Build history of the part. All positions in model axes, mm. A direction names the side the tool comes from. Give positions to 0.01 mm unless a question says otherwise; leave off trailing zeros. Order: outer loops, then holes, each group sorted by start corner. A loop starts at its lowest first (then second) coordinate and runs counter-clockwise, first axis right, second up. Notation, with made-up numbers: (-16.5, 83) - (-0.5, 83) arc R31 cw to (-0.5, 107) - close; hole circle Ø11 at (38.25, 75.5). An arc over 180 degrees is marked (long way). Use a Markdown table: item, result.
from build123d import *

# Parameters (mm, degrees)
SKETCH_1_W           = 90
SKETCH_1_H           = 50
EXTRUDE_1_DEPTH      = 10
CUT_EXTRUDE_2_DEPTH  = 5
SKETCH_7_R           = 1.6
CUT_EXTRUDE_3_DEPTH  = 10
MIRROR_3_DEPTH       = 10
MIRROR_START         = 5
MIRROR_3_2_OUTLINE_R = 1.6
MIRROR_3_2_DEPTH     = 5
SKETCH_8_R           = 5
EXTRUDE_2_DEPTH      = 30
SKETCH_10_W          = 35
SKETCH_10_H          = 20.2
EXTRUDE_6_DEPTH      = 5
SKETCH_11_W          = 102.2
SKETCH_11_H          = 51.5
CUT_EXTRUDE_4_DEPTH  = 6
SKETCH_12_W          = 7.5
SKETCH_12_H          = 13.7
CUT_EXTRUDE_5_DEPTH  = 50
FILLET_2_R           = 5
CUT_EXTRUDE_6_DEPTH  = 15
CUT_EXTRUDE_7_DEPTH  = 10
SKETCH_15_R          = 5
EXTRUDE_7_DEPTH      = 10
SKETCH_16_R          = 2
CUT_EXTRUDE_8_DEPTH  = 10
SKETCH_17_R          = 1.6
CUT_EXTRUDE_9_DEPTH  = 10


# Read off the part's stored shape, not the designer's step: Зеркальное отражение3
with BuildPart() as part:
    # Эскиз1 → Бобышка-Вытянуть1 (new body)
    with BuildSketch(Plane(origin=(0, 0, 0), x_dir=(1, 0, 0), z_dir=(0, 1, 0))):
        with Locations((4.158751696, -0.305291723)):
            Rectangle(SKETCH_1_W, SKETCH_1_H)
    extrude(amount=EXTRUDE_1_DEPTH)

    # Эскиз2 → Вырез-Вытянуть2 (cut)
    with BuildSketch(Plane.XZ):
        Polygon((-40.841248304, 14.557268649), (-23.163578774, -3.12040088), (-12.4155557, 7.627622194), (-30.09322523, 25.305291723), (-40.841248304, 25.305291723), align=None)
    extrude(amount=-CUT_EXTRUDE_2_DEPTH, mode=Mode.SUBTRACT)

    # Эскиз7 → Вырез-Вытянуть3 (cut)
    with BuildSketch(Plane.XZ.offset(-5)):
        with Locations(Location((-31.931702861, 16.39574628, 0), (0, 0, 270))):
            Circle(SKETCH_7_R)
        with Locations(Location((-23.446421487, 7.910464906, 0), (0, 0, 270))):
            Circle(SKETCH_7_R)
    extrude(amount=-CUT_EXTRUDE_3_DEPTH, mode=Mode.SUBTRACT)

    # Зеркальное отражение3 outline → Зеркальное отражение3 (add)
    with BuildSketch(Plane(origin=(0, 0, 0), x_dir=(1, 0, 0), z_dir=(0, 1, 0))):
        Polygon((-40.841248304, 63.946685203), (-40.841248304, 24.694708277), (49.158751696, 24.694708277), (49.158751696, -25.305291723), (128.410728622, -25.305291723), (110.733059092, -7.627622194), (121.481082166, 3.12040088), (139.158751696, -14.557268649), (139.158751696, 63.946685203), (121.481082166, 46.269015673), (110.733059092, 57.017038747), (128.410728622, 74.694708277), (-30.09322523, 74.694708277), (-12.4155557, 57.017038747), (-23.163578774, 46.269015673), align=None)
    extrude(amount=MIRROR_3_DEPTH)

    # Mirror 3 2 outline → Mirror 3 2 (add)
    # profile 1 of 3: a face of its own
    with BuildSketch(Plane(origin=(0, 0, 0), x_dir=(1, 0, 0), z_dir=(0, 1, 0)).offset(MIRROR_START)):
        Polygon((-40.841248304, 74.694708277), (-40.841248304, 63.946685203), (-23.163578774, 46.269015673), (-12.4155557, 57.017038747), (-30.09322523, 74.694708277), align=None)
        with Locations((-23.446421487, 57.29988146)):
            Circle(MIRROR_3_2_OUTLINE_R, mode=Mode.SUBTRACT)
        with Locations((-31.931702861, 65.785162834)):
            Circle(MIRROR_3_2_OUTLINE_R, mode=Mode.SUBTRACT)
    # profile 2 of 3: a face of its own
    with BuildSketch(Plane(origin=(0, 0, 0), x_dir=(1, 0, 0), z_dir=(0, 1, 0)).offset(MIRROR_START)):
        Polygon((110.733059092, -7.627622194), (128.410728622, -25.305291723), (139.158751696, -25.305291723), (139.158751696, -14.557268649), (121.481082166, 3.12040088), align=None)
        with Locations((130.249206253, -16.39574628)):
            Circle(MIRROR_3_2_OUTLINE_R, mode=Mode.SUBTRACT)
        with Locations((121.763924879, -7.910464906)):
            Circle(MIRROR_3_2_OUTLINE_R, mode=Mode.SUBTRACT)
    # profile 3 of 3: a face of its own
    with BuildSketch(Plane(origin=(0, 0, 0), x_dir=(1, 0, 0), z_dir=(0, 1, 0)).offset(MIRROR_START)):
        Polygon((139.158751696, 74.694708277), (128.410728622, 74.694708277), (110.733059092, 57.017038747), (121.481082166, 46.269015673), (139.158751696, 63.946685203), align=None)
        with Locations((121.763924879, 57.29988146)):
            Circle(MIRROR_3_2_OUTLINE_R, mode=Mode.SUBTRACT)
        with Locations((130.249206253, 65.785162834)):
            Circle(MIRROR_3_2_OUTLINE_R, mode=Mode.SUBTRACT)
    extrude(amount=MIRROR_3_2_DEPTH)

    # Эскиз8 → Бобышка-Вытянуть2 (add)
    with BuildSketch(Plane(origin=(0, 10, 0), x_dir=(1, 0, 0), z_dir=(0, 1, 0))):
        with Locations(Location((49.158751696, 46.794708277, 0), (0, 0, 90))):
            Circle(SKETCH_8_R)
        with Locations(Location((94.158751696, 46.794708277, 0), (0, 0, 90))):
            Circle(SKETCH_8_R)
        with Locations(Location((94.158751696, 2.594708277, 0), (0, 0, 90))):
            Circle(SKETCH_8_R)
        with Locations(Location((4.158751696, 2.594708277, 0), (0, 0, 90))):
            Circle(SKETCH_8_R)
        with Locations(Location((49.158751696, 2.594708277, 0), (0, 0, 90))):
            Circle(SKETCH_8_R)
        with Locations(Location((4.158751696, 46.794708277, 0), (0, 0, 90))):
            Circle(SKETCH_8_R)
    extrude(amount=EXTRUDE_2_DEPTH)

    # Эскиз10 → Бобышка-Вытянуть6 (add)
    with BuildSketch(Plane(origin=(0, 40, 0), x_dir=(1, 0, 0), z_dir=(0, 1, 0))):
        Polygon((9.158751696, 51.794708277), (9.158751696, 39.794708277), (44.158751696, 39.794708277), (44.158751696, 51.794708277), (54.158751696, 51.794708277), (54.158751696, 39.794708277), (89.158751696, 39.794708277), (89.158751696, 51.794708277), (99.158751696, 51.794708277), (99.158751696, -2.405291723), (89.158751696, -2.405291723), (89.158751696, 9.594708277), (54.158751696, 9.594708277), (54.158751696, -2.405291723), (44.158751696, -2.405291723), (44.158751696, 9.594708277), (9.158751696, 9.594708277), (9.158751696, -2.405291723), (-0.841248304, -2.405291723), (-0.841248304, 51.794708277), align=None)
        with Locations((26.658751696, 24.694708277)):
            Rectangle(SKETCH_10_W, SKETCH_10_H, mode=Mode.SUBTRACT)
        with Locations((71.658751696, 24.694708277)):
            Rectangle(SKETCH_10_W, SKETCH_10_H, mode=Mode.SUBTRACT)
    extrude(amount=EXTRUDE_6_DEPTH)

    # Эскиз11 → Вырез-Вытянуть4 (cut)
    with BuildSketch(Plane(origin=(0, 0, 0), x_dir=(-1, 0, 0), z_dir=(0, -1, 0))):
        with Locations((-47.698520167, 25.294708277)):
            Rectangle(SKETCH_11_W, SKETCH_11_H)
    extrude(amount=-CUT_EXTRUDE_4_DEPTH, mode=Mode.SUBTRACT)

    # Эскиз12 → Вырез-Вытянуть5 (cut)
    with BuildSketch(Plane(origin=(0, 10, 0), x_dir=(1, 0, 0), z_dir=(0, 1, 0))):
        with Locations((108.408751696, 24.844708277)):
            Rectangle(SKETCH_12_W, SKETCH_12_H)
    extrude(amount=-CUT_EXTRUDE_5_DEPTH, mode=Mode.SUBTRACT)

    # Скругление2
    fillet_2_edges = [part.edges().sort_by_distance(p)[0] for p in [
        (54.158751696, 42.5, -9.594708277),
        (9.158751696, 42.5, -9.594708277),
        (-0.841248304, 42.5, 2.405291723),
        (9.158751696, 42.5, 2.405291723),
        (44.158751696, 42.5, -9.594708277),
        (54.158751696, 42.5, 2.405291723),
        (44.158751696, 42.5, 2.405291723),
        (89.158751696, 42.5, -9.594708277),
        (89.158751696, 42.5, 2.405291723),
        (99.158751696, 42.5, 2.405291723),
        (54.158751696, 42.5, -39.794708277),
        (9.158751696, 42.5, -39.794708277),
        (44.158751696, 42.5, -39.794708277),
        (99.158751696, 42.5, -51.794708277),
        (89.158751696, 42.5, -39.794708277),
        (89.158751696, 42.5, -51.794708277),
        (54.158751696, 42.5, -51.794708277),
        (44.158751696, 42.5, -51.794708277),
        (9.158751696, 42.5, -51.794708277),
        (-0.841248304, 42.5, -51.794708277),
    ]]
    fillet(fillet_2_edges, radius=FILLET_2_R - 0.0001)  # a hair under: the kernel refuses the full size

    # Эскиз13 → Вырез-Вытянуть6 (cut)
    with BuildSketch(Plane.XZ):
        Polygon((-15.09322523, 25.305291723), (2.5844443, 7.627622194), (95.733059092, 7.627622194), (113.410728622, 25.305291723), align=None)
        Polygon((-40.841248304, -0.442731351), (-23.163578774, -18.12040088), (-23.163578774, -31.269015673), (-40.841248304, -48.946685203), align=None)
        Polygon((-15.09322523, -74.694708277), (2.5844443, -57.017038747), (95.733059092, -57.017038747), (113.410728622, -74.694708277), align=None)
        Polygon((139.158751696, -0.442731351), (121.481082166, -18.12040088), (121.481082166, -31.269015673), (139.158751696, -48.946685203), align=None)
    extrude(amount=-CUT_EXTRUDE_6_DEPTH, mode=Mode.SUBTRACT)

    # Эскиз14 → Вырез-Вытянуть7 (cut)
    with BuildSketch(Plane.XZ.offset(-6)):
        Polygon((4.598520167, -9.023164144), (4.598520167, -40.56625241), (41.357986916, -24.794708277), align=None)
        Polygon((13.833681258, -7.544708277), (47.698520167, -22.074320609), (81.563359076, -7.544708277), align=None)
        Polygon((13.833681258, -42.044708277), (47.698520167, -27.515095944), (81.563359076, -42.044708277), align=None)
        Polygon((54.039053419, -24.794708277), (90.798520167, -40.56625241), (90.798520167, -9.023164144), align=None)
    extrude(amount=-CUT_EXTRUDE_7_DEPTH, mode=Mode.SUBTRACT)

    # Эскиз15 → Бобышка-Вытянуть7 (add)
    with BuildSketch(Plane.XZ):
        with Locations((49.158751696, 7.627622194)):
            Circle(SKETCH_15_R)
        with Locations((-23.163578774, -24.694708277)):
            Circle(SKETCH_15_R)
        with Locations((121.481082166, -24.694708277)):
            Circle(SKETCH_15_R)
        with Locations((49.158751696, -57.017038747)):
            Circle(SKETCH_15_R)
    extrude(amount=-EXTRUDE_7_DEPTH)

    # Эскиз16 → Вырез-Вытянуть8 (cut)
    with BuildSketch(Plane.XZ):
        with Locations(Location((49.158751696, 7.627622194, 0), (0, 0, 270))):
            Circle(SKETCH_16_R)
        with Locations(Location((-23.163578774, -24.694708277, 0), (0, 0, 270))):
            Circle(SKETCH_16_R)
        with Locations(Location((121.481082166, -24.694708277, 0), (0, 0, 270))):
            Circle(SKETCH_16_R)
        with Locations(Location((49.158751696, -57.017038747, 0), (0, 0, 270))):
            Circle(SKETCH_16_R)
    extrude(amount=-CUT_EXTRUDE_8_DEPTH, mode=Mode.SUBTRACT)

    # Эскиз17 → Вырез-Вытянуть9 (cut)
    with BuildSketch(Plane(origin=(0, 45, 0), x_dir=(1, 0, 0), z_dir=(0, 1, 0))):
        with Locations(Location((4.158751696, 34.74175422, 0), (0, 0, 270))):
            Circle(SKETCH_17_R)
        with Locations(Location((94.158751696, 34.794708277, 0), (0, 0, 270))):
            Circle(SKETCH_17_R)
        with Locations(Location((94.158751696, 14.594708277, 0), (0, 0, 270))):
            Circle(SKETCH_17_R)
        with Locations(Location((4.158751696, 14.594708277, 0), (0, 0, 270))):
            Circle(SKETCH_17_R)
    extrude(amount=-CUT_EXTRUDE_9_DEPTH, mode=Mode.SUBTRACT)


solid = part.part
1) Two-plate mould, pull along Y, no slides. Class faces 5 (the flat face through (-31.879, 2.465, -54.984)), 6 (the flat face through (-27, 5, 11)), 7 (the flat face through (50, 40, -25)): +Y half, -Y half, draft (parallel to the pull), parting line (faces both ways), or undercut.
Computed:
| item | result |
|---|---|
| face 5 | draft |
| face 6 | -Y half |
| face 7 | undercut |
2) Slice it at A-A (x = 56.5). Write the cut outline in (y, z), and give its area (3 significant figures).
Computed:
| item | result |
|---|---|
| outline | (0, -57.02) - (10, -57.02) - (10, -42.04) - (6, -42.04) - (6, -51.04) - (0, -51.04) - close; (0, 0.46) - (6, 0.46) - (6, -7.54) - (10, -7.54) - (10, 7.63) - (0, 7.63) - close; (6, -31.29) - (10, -31.29) - (10, -25.85) - (6, -25.85) - close; (6, -23.74) - (10, -23.74) - (10, -18.3) - (6, -18.3) - close; (40, -40.56) - (45, -40.56) - (45, -34.79) - (40, -34.79) - close; (40, -14.59) - (45, -14.59) - (45, -8.83) - (40, -8.83) - close |
| area | 301 mm² |
3) Wall check: line 1 (Z direction, x = 71, y = 9); line 2 (X direction, y = 12, z = -3); line 3 (Z direction, x = -26.5, y = 7). Give the ranges that are in metal, low to high. Write a range as from..to.
Computed:
| item | result |
|---|---|
| line 1 | z = -57.02..-42.04, -37.51..-32.07, -17.52..-12.08, -7.54..7.63 |
| line 2 | x = -0.82..9.14, 44.18..54.14, 89.18..99.14 |
| line 3 | z = -74.69..-34.61, -28.42..-20.97, -14.78..25.31 |
4) Slice it at B-B (y = 27). Write the cut outline in (x, z).
Computed:
| item | result |
|---|---|
| outline | circle Ø10 at (4.16, -46.79); circle Ø10 at (4.16, -2.59); circle Ø10 at (49.16, -46.79); circle Ø10 at (49.16, -2.59); circle Ø10 at (94.16, -46.79); circle Ø10 at (94.16, -2.59) |
5) Pin check, flat tips, straight feed: P1, Ø8, axis at y = 2.5, z = -27.5, coming from the -X side; P2, Ø6.5, axis at x = 58, y = 3.5, coming from the +Z side; P3, Ø1.5, axis at x = 96, z = -1.5, coming from the -Y side. Stop position of each tip, or through.
Computed:
| item | result |
|---|---|
| P1 | stops at x = -28.16 |
| P2 | stops at z = 7.63 |
| P3 | stops at y = 6 |
6) Tool access for faces 1 (the flat face through (-17.71, 2.46, -51.72)), 2 (the cylindrical face through (42.655, 42.535, -8.169)), 3 (the cylindrical face through (51.074, 24.79, -51.413)), 4 (the flat face through (26, 42, -39.795)): list every direction of +Z, -Z, +X, -X, +Y, -Y with a clear straight run to the whole face (end or side of a thin tool).
Computed:
| item | result |
|---|---|
| face 1 | -Y |
| face 2 | +Z, +Y |
| face 3 | none |
| face 4 | -Z, +Y |
